```python
from build123d import *

# Parameters (mm, degrees)
SKETCH1_W           = 120
SKETCH1_H           = 40
BOSS_EXTRUDE1_DEPTH = 5
SKETCH2_R           = 4.05
SKETCH2_R_2         = 3.05
CUT_EXTRUDE1_DEPTH  = 64.442887702
FILLET1_R           = 10


with BuildPart() as part:
    # Sketch1 → Boss-Extrude1 (new body)
    with BuildSketch(Plane(origin=(0, 0, 0), x_dir=(1, 0, 0), z_dir=(0, 1, 0))):
        Rectangle(SKETCH1_W, SKETCH1_H)
    extrude(amount=BOSS_EXTRUDE1_DEPTH)

    # Sketch2 → Cut-Extrude1 (cut, through all)
    with BuildSketch(Plane(origin=(0, 5, 0), x_dir=(1, 0, 0), z_dir=(0, 1, 0))):
        with Locations(Location((-25, 0, 0), (0, 0, 270))):
            Circle(SKETCH2_R)
        with Locations(Location((-50, 0, 0), (0, 0, 270))):
            Circle(SKETCH2_R_2)
    cut_extrude1 = extrude(amount=-CUT_EXTRUDE1_DEPTH, mode=Mode.SUBTRACT)

    # Mirror1: Cut-Extrude1 across plane
    add(cut_extrude1.mirror(Plane(origin=(0, 0, 0), x_dir=(0, 0, 1), z_dir=(1, 0, 0))), mode=Mode.SUBTRACT)

    # Fillet1
    fillet1_edges = [part.edges().sort_by_distance(p)[0] for p in [
        (60, 2.5, 20),
        (-60, 2.5, 20),
        (-60, 2.5, -20),
        (60, 2.5, -20),
    ]]
    fillet(fillet1_edges, radius=FILLET1_R)


solid = part.part
```
Source: CAD feature listing. Evaluate the final solid. Frame: model axes, mm. Coordinates: 2 decimals unless noted, no trailing zeros. Loops run counter-clockwise (first coordinate to the right, second up) from the corner with the lowest first, then second, coordinate; pieces in that order, holes last. Notation, with made-up numbers: M 37.25,65.25 L 62.25,65.25 A17 ccw 62.25,86.25 Z; hole C 1.5,-15.5 d11. An arc over 180 degrees is marked long. Use a Markdown table: item, result. Add a question column.
Q1. First-contact query: pin 1 (2 mm diameter, centred on y = 3.5, z = 12, fed in from -X). Flat tip, straight axial feed; report the tip coordinate or a pass-through.
Q2. Section query A-A, the plane z = 0. Return loops of the section in (x, y).
Q3. Section query B-B, the plane y = 1.5. Return loops of the section in (x, z), and give its area (3 significant figures).
Q4. Material intervals for L1, parallel to X at y = 1.95, z = 0; L2, parallel to X at y = 1.7, z = 1; L3, parallel to X at y = 2.05, z = -13.5, sorted ascending.
Q5. Draft query along Z for faces 1 (the cylindrical face through (-52.977, 2.535, -0.661)), 2 (the cylindrical face through (56.99, 2.54, 17.15)), 3 (the cylindrical face through (-57.15, 2.54, -16.99)). Return one class per face: pulls with the +Z half, pulls with the -Z half, needs draft (parallel to the pull), parting line crosses it, or undercut.
Q6. Section query C-C, the plane x = -25. Return loops of the section in (y, z), and give its area (4 significant figures).
Q7. Section query D-D, the plane z = 15.5. Return loops of the section in (x, y), and give its area (3 significant figures).
Result:
| question | item | result |
|---|---|---|
| 1 | pin 1 | stops at x = -59.95 |
| 2 | outline | M -60,0 L -53.05,0 L -53.05,5 L -60,5 Z; M -46.95,0 L -29.05,0 L -29.05,5 L -46.95,5 Z; M -20.95,0 L 20.95,0 L 20.95,5 L -20.95,5 Z; M 29.05,0 L 46.95,0 L 46.95,5 L 29.05,5 Z; M 53.05,0 L 60,0 L 60,5 L 53.05,5 Z |
| 3 | outline | M -60,-10 A10 ccw -50,-20 L 50,-20 A10 ccw 60,-10 L 60,10 A10 ccw 50,20 L -50,20 A10 ccw -60,10 Z; hole C -50,0 d6.1; hole C -25,0 d8.1; hole C 25,0 d8.1; hole C 50,0 d6.1 |
| 3 | area | 4,550 mm2 |
| 4 | L1 | x = -60 to -53.05, -46.95 to -29.05, -20.95 to 20.95, 29.05 to 46.95, 53.05 to 60 |
| 4 | L2 | x = -60 to -52.88, -47.12 to -28.92, -21.08 to 21.08, 28.92 to 47.12, 52.88 to 60 |
| 4 | L3 | x = -59.37 to 59.37 |
| 5 | face 1 | undercut |
| 5 | face 2 | pulls with the +Z half |
| 5 | face 3 | pulls with the -Z half |
| 6 | outline | M 0,-20 L 5,-20 L 5,-4.05 L 0,-4.05 Z; M 0,4.05 L 5,4.05 L 5,20 L 0,20 Z |
| 6 | area | 159.5 mm2 |
| 7 | outline | M -58.35,0 L 58.35,0 L 58.35,5 L -58.35,5 Z |
| 7 | area | 584 mm2 |
